Geometry check sheet. Reference: the model listing, model coordinates, mm. A direction names the side the tool comes from. Round coordinates to 2 decimals unless told otherwise and drop trailing zeros. Write each loop counter-clockwise with the first axis right and the second up, starting at its lowest first coordinate (ties: lowest second). Pieces come first, ordered by that corner, then holes. Notation, with made-up numbers: (51.25, 79) -> (93.25, 79) arc R32 ccw to (93.25, 115) -> close; hole circle Ø7 at (-32, 88). An arc over 180 degrees is marked (long way). Return JSON: item names as keys, results as strings. Group by question number.
from build123d import *

# Parameters (mm, degrees)
SKETCH1_R           = 4.95
BOSS_EXTRUDE1_DEPTH = 13.8
SKETCH2_R           = 6
BOSS_EXTRUDE2_DEPTH = 19.1
SKETCH7_R           = 2.65
CUT_EXTRUDE1_DEPTH  = 33.9
CHAMFER1_SIZE       = 0.4


with BuildPart() as part:
    # Sketch1 → Boss-Extrude1 (new body)
    with BuildSketch(Plane(origin=(0, 0, 0), x_dir=(1, 0, 0), z_dir=(0, 1, 0))):
        Circle(SKETCH1_R)
    extrude(amount=BOSS_EXTRUDE1_DEPTH)

    # Sketch2 → Boss-Extrude2 (add)
    with BuildSketch(Plane(origin=(0, 13.8, 0), x_dir=(1, 0, 0), z_dir=(0, 1, 0))):
        Circle(SKETCH2_R)
    extrude(amount=BOSS_EXTRUDE2_DEPTH)

    # Sketch7 → Cut-Extrude1 (cut, through all)
    with BuildSketch(Plane(origin=(0, 0, 0), x_dir=(1, 0, 0), z_dir=(0, 1, 0))):
        Circle(SKETCH7_R)
    extrude(amount=CUT_EXTRUDE1_DEPTH, mode=Mode.SUBTRACT)

    # Chamfer1
    chamfer1_edges = [part.edges().sort_by_distance(p)[0] for p in [
        (-2.65, 0, 0),
    ]]
    chamfer(chamfer1_edges, length=CHAMFER1_SIZE)


solid = part.part
1) Sectioned sample at C-C on y = 19.5. Enter the section's corners in (x, z).
2) Sectioned sample at A-A on x = 0. Enter the section's corners in (y, z), and give its area (3 significant figures).
3) Tool access check on faces 1 (the face through (3, 32.9, 1)), 2 (the face through (4.72, 6.8, -1.49)). Record the directions out of +Z, -Z, +X, -X, +Y, -Y that give a thin tool (end or side, any length) a straight path to the whole face; none if there is none.
4) Sectioned sample at D-D on z = -4.5. Enter the section's corners in (x, y).
5) Go/stop test with flat-tipped pins: P1, Ø3, axis at y = 27, z = -3.5, coming from the +X side; P2, Ø2, axis at x = 4, y = 12, coming from the +Z side; P3, Ø1, axis at y = 13, z = -1, coming from the -X side. Record where each tip stops, or that it passes through.
6) Material ranges on probe 1 along Z at (x, y) = (0, 25); probe 2 along Z at (x, y) = (0, 12.5), recorded low to high. Write a range as [from, to].
7) Sectioned sample at B-B on z = 0. Enter the section's corners in (x, y).
8) Mould release check, pull along X, two halves, no side actions. Record for faces 3 (the face through (-1.36, 13.8, -4.92)), 4 (the face through (2.45, 16.42, 1.01)), 5 (the face through (-6, 23, 0)): +X half, -X half, draft (parallel to the pull), parting line (faces both ways), or undercut.
Evaluation:
{
 "1": {"outline": "circle Ø12 at (0, 0); hole circle Ø5.3 at (0, 0)"},
 "2": {"outline": "(0, -4.95) -> (13.8, -4.95) -> (13.8, -6) -> (32.9, -6) -> (32.9, -2.65) -> (0.4, -2.65) -> (0, -3.05) -> close; (0, 3.05) -> (0.4, 2.65) -> (32.9, 2.65) -> (32.9, 6) -> (13.8, 6) -> (13.8, 4.95) -> (0, 4.95) -> close", "area": "191 mm2"},
 "3": {"face 1": "+Z, -Z, +X, -X, +Y", "face 2": "-Y"},
 "4": {"outline": "(-3.97, 13.8) -> (-2.06, 13.8) -> (-2.06, 0) -> (2.06, 0) -> (2.06, 13.8) -> (3.97, 13.8) -> (3.97, 32.9) -> (-3.97, 32.9) -> close"},
 "5": {"P1": "stops at x = 5.66", "P2": "stops at z = 3.94", "P3": "stops at x = -4.92"},
 "6": {"probe 1": "z = [-6, -2.65], [2.65, 6]", "probe 2": "z = [-4.95, -2.65], [2.65, 4.95]"},
 "7": {"outline": "(-6, 13.8) -> (-4.95, 13.8) -> (-4.95, 0) -> (-3.05, 0) -> (-2.65, 0.4) -> (-2.65, 32.9) -> (-6, 32.9) -> close; (2.65, 0.4) -> (3.05, 0) -> (4.95, 0) -> (4.95, 13.8) -> (6, 13.8) -> (6, 32.9) -> (2.65, 32.9) -> close"},
 "8": {"face 3": "draft", "face 4": "undercut", "face 5": "parting line"}
}
